Model file for the job. Use its own axes, mm. Coordinates: 2 decimals unless noted, no trailing zeros. Order: outer loops, then holes, each group sorted by start corner. A loop starts at its lowest first (then second) coordinate and runs counter-clockwise, first axis right, second up. Notation, with made-up numbers: (-35.5, 9.25) -> (-12.5, 9.25) arc R15 cw to (-12.5, 19.25) -> close; hole circle Ø2 at (19, -16). An arc over 180 degrees is marked (long way). Write item = value, one per line. Start each with the question number.
Q1. Wall check: line 1 (Y direction, x = 72, z = 3.5); line 2 (X direction, y = -5.25, z = 3.8); line 3 (X direction, y = 6.5, z = 5.7). Give the ranges that are in metal, low to high. Write a range as from..to.
Q2. Cut at B-B, the plane x = -13.5. List the corners of the cut face in (y, z).
Q3. Cut at C-C, the plane x = 34.5. List the corners of the cut face in (y, z), plus the area to 3 significant figures.
Q4. Cut at A-A, the plane x = -81.5. List the corners of the cut face in (y, z), plus the area to 3 significant figures.
Q5. Flat gauge pins, fed straight in: pin 1 (2 mm diameter, centred on x = -13.5, z = 3.5, fed in from +Y); pin 2 (1 mm diameter, centred on x = -27, z = 3.5, fed in from -Y). Where does each tip first touch, or does it go through?
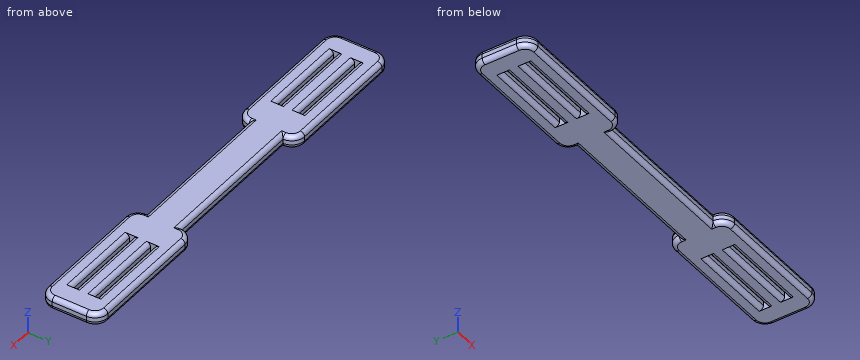
from build123d import *

# Parameters (mm, degrees)
BOX003_W     = 40
BOX003_H     = 2
BOX003_DEPTH = 10
BOX004_W     = 40
BOX004_H     = 2
BOX004_DEPTH = 10
BOX002_W     = 40
BOX002_H     = 2
BOX002_DEPTH = 10
BOX005_W     = 70
BOX005_H     = 6
BOX005_DEPTH = 10
BOX006_W     = 70
BOX006_H     = 6
BOX006_DEPTH = 10
BOX001_W     = 40
BOX001_H     = 2
BOX001_DEPTH = 10
BOX_W        = 200
BOX_H        = 28
BOX_DEPTH    = 6
FILLET_R     = 5.99
FILLET001_R  = 2


with BuildPart() as cube003:
    # Box003 → Box003 (new body)
    with BuildSketch(Plane(origin=(40, -6, 0), x_dir=(1, 0, 0), z_dir=(0, 0, 1))):
        with Locations((20, 1)):
            Rectangle(BOX003_W, BOX003_H)
    extrude(amount=BOX003_DEPTH)


with BuildPart() as cube004:
    # Box004 → Box004 (new body)
    with BuildSketch(Plane(origin=(40, 4, 0), x_dir=(1, 0, 0), z_dir=(0, 0, 1))):
        with Locations((20, 1)):
            Rectangle(BOX004_W, BOX004_H)
    extrude(amount=BOX004_DEPTH)


with BuildPart() as cube002:
    # Box002 → Box002 (new body)
    with BuildSketch(Plane(origin=(-100, 4, 0), x_dir=(1, 0, 0), z_dir=(0, 0, 1))):
        with Locations((20, 1)):
            Rectangle(BOX002_W, BOX002_H)
    extrude(amount=BOX002_DEPTH)


with BuildPart() as cube005:
    # Box005 → Box005 (new body)
    with BuildSketch(Plane(origin=(-45, -14, 0), x_dir=(1, 0, 0), z_dir=(0, 0, 1))):
        with Locations((35, 3)):
            Rectangle(BOX005_W, BOX005_H)
    extrude(amount=BOX005_DEPTH)


with BuildPart() as cube006:
    # Box006 → Box006 (new body)
    with BuildSketch(Plane(origin=(-45, 8, 0), x_dir=(1, 0, 0), z_dir=(0, 0, 1))):
        with Locations((35, 3)):
            Rectangle(BOX006_W, BOX006_H)
    extrude(amount=BOX006_DEPTH)


with BuildPart() as holes:
    # Box001 → Box001 (new body)
    with BuildSketch(Plane(origin=(-100, -6, 0), x_dir=(1, 0, 0), z_dir=(0, 0, 1))):
        with Locations((20, 1)):
            Rectangle(BOX001_W, BOX001_H)
    extrude(amount=BOX001_DEPTH)

    # Fusion: union Cube003, Cube004, Cube002, Cube005, Cube006
    add(cube003.part)
    add(cube004.part)
    add(cube002.part)
    add(cube005.part)
    add(cube006.part)


with BuildPart() as fillet001:
    # Box → Box (new body)
    with BuildSketch(Plane(origin=(-110, -14, 0), x_dir=(1, 0, 0), z_dir=(0, 0, 1))):
        with Locations((100, 14)):
            Rectangle(BOX_W, BOX_H)
    extrude(amount=BOX_DEPTH)

    # Cut: cut Holes
    add(holes.part, mode=Mode.SUBTRACT)

    # Fillet
    fillet_edges = [fillet001.edges().sort_by_distance(p)[0] for p in [
        (-110, -14, 3),
        (-110, 14, 3),
        (-45, -14, 3),
        (-45, 14, 3),
        (25, 14, 3),
        (90, 14, 3),
        (90, -14, 3),
        (25, -14, 3),
    ]]
    fillet(fillet_edges, radius=FILLET_R)

    # Fillet001
    fillet001_edges = [fillet001.edges().sort_by_distance(p)[0] for p in [
        (-110, 0, 6),
        (-110, 0, 0),
        (-77.5, 14, 6),
        (-108.24557, 12.24557, 6),
        (-46.75443, 12.24557, 6),
        (-108.24557, -12.24557, 6),
        (-10, 8, 6),
        (-77.5, -14, 6),
        (-46.75443, -12.24557, 6),
        (26.75443, 12.24557, 6),
        (57.5, 14, 6),
        (-10, -8, 6),
        (88.24557, 12.24557, 6),
        (90, 0, 6),
        (26.75443, -12.24557, 6),
        (88.24557, -12.24557, 6),
        (57.5, -14, 6),
        (-80, -6, 6),
        (-80, -4, 6),
        (-80, 4, 6),
        (-80, 6, 6),
        (60, 4, 6),
        (60, 6, 6),
        (60, -6, 6),
        (60, -4, 6),
        (-108.24557, -12.24557, 0),
        (-108.24557, 12.24557, 0),
        (-77.5, 14, 0),
        (-46.75443, 12.24557, 0),
        (-10, 8, 0),
        (-77.5, -14, 0),
        (-46.75443, -12.24557, 0),
        (26.75443, 12.24557, 0),
        (57.5, 14, 0),
        (-10, -8, 0),
        (88.24557, 12.24557, 0),
        (90, 0, 0),
        (26.75443, -12.24557, 0),
        (88.24557, -12.24557, 0),
        (57.5, -14, 0),
        (-80, -6, 0),
        (-80, -4, 0),
        (-80, 4, 0),
        (-80, 6, 0),
        (60, 4, 0),
        (60, 6, 0),
        (60, -6, 0),
        (60, -4, 0),
    ]]
    fillet(fillet001_edges, radius=FILLET001_R)


solid = fillet001.part
Here are the results:
q1.line_1 = -14..-6, -4..4, 6..14
q1.line_2 = -110..-100, -60..40, 80..90
q1.line_3 = -109.05..-100, -60..40, 80..89.05
q2.outline = (-8, 2) arc R2 ccw to (-6, 0) -> (6, 0) arc R2 ccw to (8, 2) -> (8, 4) arc R2 ccw to (6, 6) -> (-6, 6) arc R2 ccw to (-8, 4) -> close
q3.outline = (-14, 2) arc R2 ccw to (-12, 0) -> (12, 0) arc R2 ccw to (14, 2) -> (14, 4) arc R2 ccw to (12, 6) -> (-12, 6) arc R2 ccw to (-14, 4) -> close
q3.area = 165 mm²
q4.outline = (-14, 2) arc R2 ccw to (-12, 0) -> (-8, 0) arc R2 ccw to (-6, 2) -> (-6, 4) arc R2 ccw to (-8, 6) -> (-12, 6) arc R2 ccw to (-14, 4) -> close; (-4, 2) arc R2 ccw to (-2, 0) -> (2, 0) arc R2 ccw to (4, 2) -> (4, 4) arc R2 ccw to (2, 6) -> (-2, 6) arc R2 ccw to (-4, 4) -> close; (6, 2) arc R2 ccw to (8, 0) -> (12, 0) arc R2 ccw to (14, 2) -> (14, 4) arc R2 ccw to (12, 6) -> (8, 6) arc R2 ccw to (6, 4) -> close
q4.area = 134 mm²
q5.pin_1 = 8
q5.pin_2 = -8
